Geometry check sheet. Reference: the model listing, model coordinates, mm. Face numbers are marked on the shaded views. A direction names the side the tool comes from. Coordinates: 2 decimals unless noted, no trailing zeros. Order: outer loops, then holes, each group sorted by start corner. A loop starts at its lowest first (then second) coordinate and runs counter-clockwise, first axis right, second up. Notation, with made-up numbers: M 87.5,-23 L 129.5,-23 A26 cw 129.5,-9 Z; hole C 86.5,57.25 d9. An arc over 180 degrees is marked long. One line per item, written item: value. Start each with the question number.
1) Sectioned sample at A-A, the plane y = -14. Enter the section's corners in (x, z), then the cut area to 3 significant figures.
2) Go/stop test with flat-tipped pins: P1, Ø2.5, axis at y = -14, z = 9.5, coming from the -X side; P2, Ø4.5, axis at x = 3.11, y = 5.39, coming from the +Z side; P3, Ø7.5, axis at x = -13.5, z = 8.5, coming from the -Y side. Record where each tip stops, or that it passes through.
3) Sectioned sample at C-C, the plane z = 15. Enter the section's corners in (x, y), then the cut area to 3 significant figures.
4) Sectioned sample at B-B, the plane x = -14.5. Enter the section's corners in (y, z), then the cut area to 3 significant figures.
5) Sectioned sample at D-D, the plane y = 16. Enter the section's corners in (x, z), then the cut area to 3 significant figures.
6) Thickness scan on L1, parallel to Y at x = -22.9, z = 9.5; L2, parallel to Z at x = -14.5, y = 24.8; L3, parallel to X at y = 8.5, z = 7.5. Record the ranges inside material, lowest first. Write a range as from..to.
7) Access from +Z, -Z, +X, -X, +Y, -Y to the whole of each face (thin tool, end or side, straight path). Record for the marked faces 4, 5 and 6.
8) Draft check along X on the marked faces 1, 2 and 3. Enter one of: pulls with the +X half, pulls with the -X half, needs draft (parallel to the pull), parting line crosses it, or undercut.
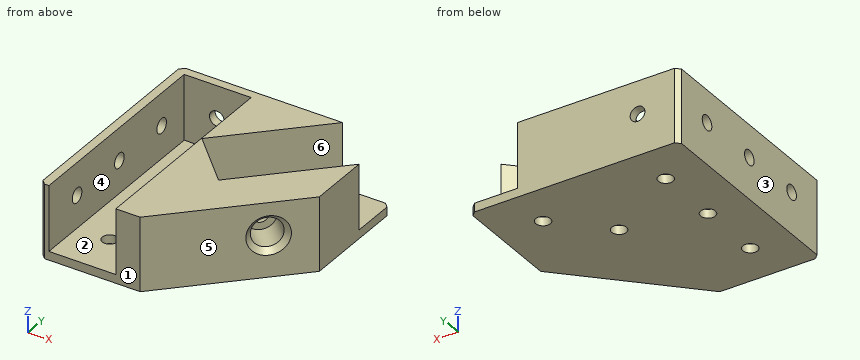
```python
from build123d import *

# Parameters (mm, degrees)
SKETCH1_W                = 48
SKETCH1_H                = 48
BOSS_EXTRUDE1_DEPTH      = 2
SKETCH2_W                = 2
SKETCH2_H                = 48
BOSS_EXTRUDE2_DEPTH      = 15
SKETCH3_W                = 48
SKETCH3_H                = 17
BOSS_EXTRUDE3_DEPTH      = 2
SKETCH6_W                = 28.6
SKETCH6_H                = 48
BOSS_EXTRUDE4_DEPTH      = 15
CUT_EXTRUDE2_DEPTH       = 15
M3_CLEARANCE_HOLE1_D     = 3.4
CHAMFER1_SIZE            = 1
CHAMFER2_SIZE            = 1
CHAMFER3_SIZE            = 1
M3_CLEARANCE_HOLE2_D     = 3.4
CHAMFER7_SIZE            = 25
M3_CLEARANCE_HOLE3_D     = 3.4
M3_CLEARANCE_HOLE3_DEPTH = 2


# Read off the part's stored shape, not the designer's step: CBORE for M3 SBHCS1
with BuildPart() as part:
    # Sketch1 → Boss-Extrude1 (new body)
    with BuildSketch(Plane.XY):
        Rectangle(SKETCH1_W, SKETCH1_H)
    extrude(amount=BOSS_EXTRUDE1_DEPTH)

    # Sketch2 → Boss-Extrude2 (add)
    with BuildSketch(Plane.XY.offset(2)):
        with Locations((-23, 0)):
            Rectangle(SKETCH2_W, SKETCH2_H)
        with Locations((-5.6, 0)):
            Rectangle(SKETCH2_W, SKETCH2_H)
    extrude(amount=BOSS_EXTRUDE2_DEPTH)

    # Sketch3 → Boss-Extrude3 (add)
    with BuildSketch(Plane(origin=(0, 24, 0), x_dir=(1, 0, 0), z_dir=(0, 1, 0))):
        with Locations((0, -8.5)):
            Rectangle(SKETCH3_W, SKETCH3_H)
    extrude(amount=BOSS_EXTRUDE3_DEPTH)

    # Sketch6 → Boss-Extrude4 (add)
    with BuildSketch(Plane.XY.offset(2)):
        with Locations((9.7, 0)):
            Rectangle(SKETCH6_W, SKETCH6_H)
    extrude(amount=BOSS_EXTRUDE4_DEPTH)

    # Sketch7 → Cut-Extrude2 (cut)
    with BuildSketch(Plane.XY.offset(17)):
        Polygon((24, 15.11055557), (4.381531726, -4.507912705), (-6.507912705, 6.381531726), (13.11055557, 26), (24, 26), align=None)
    extrude(amount=-CUT_EXTRUDE2_DEPTH, mode=Mode.SUBTRACT)

    # M3 Clearance Hole1 (through all)
    with Locations(Plane.XY.offset(2)):
        with Locations((-14.5, 16), (-14.5, 1), (-14.5, -14), (3.11055557, 5.393398282), (13.717157288, 16)):
            Hole(M3_CLEARANCE_HOLE1_D / 2)

    # Chamfer1
    chamfer1_edges = [part.edges().sort_by_distance(p)[0] for p in [
        (24, 26, 1),
    ]]
    chamfer(chamfer1_edges, length=CHAMFER1_SIZE)

    # Chamfer2
    chamfer2_edges = [part.edges().sort_by_distance(p)[0] for p in [
        (-24, 26, 8.5),
    ]]
    chamfer(chamfer2_edges, length=CHAMFER2_SIZE)

    # Chamfer3
    chamfer3_edges = [part.edges().sort_by_distance(p)[0] for p in [
        (-24, -24, 8.5),
    ]]
    chamfer(chamfer3_edges, length=CHAMFER3_SIZE)

    # M3 Clearance Hole2 (through all)
    with Locations(Plane(origin=(0, 24, 0), x_dir=(-1, 0, 0), z_dir=(0, -1, 0))):
        with Locations((14.5, -9.5)):
            Hole(M3_CLEARANCE_HOLE2_D / 2)

    # Chamfer7
    chamfer7_edges = [part.edges().sort_by_distance(p)[0] for p in [
        (24, -24, 8.5),
    ]]
    chamfer(chamfer7_edges, length=CHAMFER7_SIZE)

    # CBORE for M3 SBHCS1 outline → CBORE for M3 SBHCS1 (revolve, cut)
    with BuildSketch(Plane(origin=(5.428932188, 5.428932188, 9.5), x_dir=(0.707106781186549, 0.707106781186546, 0), z_dir=(0, 0, -1))):
        Polygon((0, 6.285786438), (1.7, 6.285786438), (1.7, 8.613455967), (3.35, 8.613455967), (3.35, 14.940532299), (4.5, 16.263455967), (0, 16.263455967), align=None)
    revolve(axis=Axis((5.428932188, 5.428932188, 9.5), (0.707106781186546, -0.707106781186549, 0)), mode=Mode.SUBTRACT)

    # M3 Clearance Hole3
    with Locations(Plane.ZY.offset(24)):
        with Locations((9.5, -14), (9.5, 1), (9.5, 16)):
            Hole(M3_CLEARANCE_HOLE3_D / 2, depth=M3_CLEARANCE_HOLE3_DEPTH)


solid = part.part
```
Final values:
1. outline: M -24,0 L -16.2,0 L -16.2,2 L -22,2 L -22,7.8 L -24,7.8 Z; M -24,11.2 L -22,11.2 L -22,17 L -24,17 Z; M -12.8,0 L 9,0 L 9,17 L -6.6,17 L -6.6,2 L -12.8,2 Z
1. area: 316 mm^2
2. P1: stops at x = -6.6
2. P2: stops at z = 2
2. P3: stops at y = 24
3. outline: M -24,-23 L -23,-24 L -22,-24 L -22,24 L -6.6,24 L -6.6,-24 L -1,-24 L 24,1 L 24,15.11 L 4.38,-4.51 L -6.51,6.38 L 13.11,26 L -23,26 L -24,25 Z
3. area: 861 mm^2
4. outline: M -24,0 L -15.7,0 L -15.7,2 L -24,2 Z; M -12.3,0 L -0.7,0 L -0.7,2 L -12.3,2 Z; M 2.7,0 L 14.3,0 L 14.3,2 L 2.7,2 Z; M 17.7,0 L 26,0 L 26,7.8 L 24,7.8 L 24,2 L 17.7,2 Z; M 24,11.2 L 26,11.2 L 26,17 L 24,17 Z
4. area: 103 mm^2
5. outline: M -24,0 L -16.2,0 L -16.2,2 L -22,2 L -22,7.8 L -24,7.8 Z; M -24,11.2 L -22,11.2 L -22,17 L -24,17 Z; M -12.8,0 L 12.02,0 L 12.02,2 L 3.11,2 L 3.11,17 L -6.6,17 L -6.6,2 L -12.8,2 Z; M 15.42,0 L 24,0 L 24,2 L 15.42,2 Z
5. area: 251 mm^2
6. L1: y = -24..-15.7, -12.3..-0.7, 2.7..14.3, 17.7..26
6. L2: z = 0..7.8, 11.2..17
6. L3: x = -24..-22, -6.6..-4.39, 17.39..24
7. face 4: +Z, -Y
7. face 5: +Z, -Z, +X, -Y
7. face 6: +Z
8. face 1: needs draft
8. face 2: undercut
8. face 3: pulls with the -X half
